```python
from build123d import *

# Parameters (mm, degrees)
EXTRUDE_1_DEPTH     = 30
CUT_EXTRUDE_1_DEPTH = 46.650848842
CUT_EXTRUDE_2_DEPTH = 46.650848842
FILLET_2_R          = 4
FILLET_3_R          = 3


with BuildPart() as part:
    # 草图1 → 凸台-拉伸1 (new body)
    with BuildSketch(Plane(origin=(0, 0, 0), x_dir=(0, 0, -1), z_dir=(1, 0, 0))):
        Polygon((0, 0), (0, -17.457543398), (0, -28), (3.576042669, -28), (20, -28), (20, -26), (3.746159887, -26), (2, -26), (2, -18.350485623), (2, 0), align=None)
    extrude(amount=EXTRUDE_1_DEPTH)

    # 草图3 → 切除-拉伸1 (cut, through all)
    with BuildSketch(Plane.XY):
        with BuildLine():
            Line((4, -12.5), (26, -12.5))
            ThreePointArc((26, -12.5), (28, -14.5), (26, -16.5))
            Line((26, -16.5), (4, -16.5))
            ThreePointArc((4, -16.5), (2, -14.5), (4, -12.5))
        make_face()
        with BuildLine():
            Line((4, -4.5), (26, -4.5))
            ThreePointArc((26, -4.5), (28, -6.5), (26, -8.5))
            Line((26, -8.5), (4, -8.5))
            ThreePointArc((4, -8.5), (2, -6.5), (4, -4.5))
        make_face()
    extrude(amount=-CUT_EXTRUDE_1_DEPTH, mode=Mode.SUBTRACT)

    # 草图4 → 切除-拉伸2 (cut, through all)
    with BuildSketch(Plane.XZ.offset(28)):
        with BuildLine():
            Line((4, -12.5), (26, -12.5))
            ThreePointArc((26, -12.5), (28.5, -15), (26, -17.5))
            Line((26, -17.5), (4, -17.5))
            ThreePointArc((4, -17.5), (1.5, -15), (4, -12.5))
        make_face()
    extrude(amount=-CUT_EXTRUDE_2_DEPTH, mode=Mode.SUBTRACT)

    # 圆角2
    fillet_2_edges = [part.edges().sort_by_distance(p)[0] for p in [
        (15, -28, 0),
    ]]
    fillet(fillet_2_edges, radius=FILLET_2_R)

    # 圆角3
    fillet_3_edges = [part.edges().sort_by_distance(p)[0] for p in [
        (15, -26, -2),
    ]]
    fillet(fillet_3_edges, radius=FILLET_3_R)


solid = part.part
```
Input: part model. Units: mm. Frame: model coordinates. A direction names the side the tool comes from. Give positions to 0.01 mm unless a question says otherwise; leave off trailing zeros. Write each loop counter-clockwise with the first axis right and the second up, starting at its lowest first coordinate (ties: lowest second). Pieces come first, ordered by that corner, then holes. Notation, with made-up numbers: (6, 74.5) - (10, 74.5) arc R22 cw to (10, 93.5) - close; hole circle Ø5 at (88, 22.25). An arc over 180 degrees is marked (long way). Write item = value, one per line. Start each with the question number.
1) Cut plane B-B (x = 5.25). Return loops of the section in (y, z).
2) Draft query along Z for faces 6 (the face through (15.21, -26.797, -1.141)), 7 (the face through (15, -16.5, -1)), 8 (the face through (15, -27, -12.5)). Return one class per face: pulls with the +Z half, pulls with the -Z half, needs draft (parallel to the pull), parting line crosses it, or undercut.
3) Cut plane A-A (z = -15). Return loops of the section in (x, y).
4) Material intervals for L1, parallel to Z at x = 8, y = -19.25; L2, parallel to Y at x = 13.25, z = -1.5; L3, parallel to Y at x = 6.5, z = -18.75, sorted ascending. Write a range as [from, to].
5) Pin query (flat end, axial travel): pin 1 (11.5 mm diameter, centred on x = 17, y = -14, fed in from -Z); pin 2 (2 mm diameter, centred on x = 20.5, z = -1, fed in from -Y); pin 3 (4.5 mm diameter, centred on x = 21.5, z = -13, fed in from +Y). Return the tip coordinate at first contact, or that it passes through.
6) Reachability of faces 1 (the face through (28, -6.5, -1)), 2 (the face through (1.5, -27, -15.1)), 3 (the face through (30, -19.1, -1.8)), 4 (the face through (0, -19.1, -1.8)), 5 (the face through (15, -26, -11)) from +Z, -Z, +X, -X, +Y, -Y: full face, straight path, thin tool, end or side. Return the list, or none.
7) Cut plane C-C (y = -14.5). Return loops of the section in (x, z).
8) Cut plane D-D (z = -11.25). Return loops of the section in (x, y), and give its area (3 significant figures).
Answers follow:
q1.outline = (-28, -20) - (-26, -20) - (-26, -17.5) - (-28, -17.5) - close; (-28, -12.5) - (-26, -12.5) - (-26, -5) arc R3 cw to (-23, -2) - (-16.5, -2) - (-16.5, 0) - (-24, 0) arc R4 ccw to (-28, -4) - close; (-12.5, -2) - (-8.5, -2) - (-8.5, 0) - (-12.5, 0) - close; (-4.5, -2) - (0, -2) - (0, 0) - (-4.5, 0) - close
q2.face_6 = pulls with the +Z half
q2.face_7 = needs draft
q2.face_8 = undercut
q3.outline = (0, -28) - (1.5, -28) - (1.5, -26) - (0, -26) - close; (28.5, -28) - (30, -28) - (30, -26) - (28.5, -26) - close
q4.L1 = [-2, 0]
q4.L2 = [-27.12, -16.5], [-12.5, -8.5], [-4.5, 0]
q4.L3 = [-28, -26]
q5.pin_1 = -2
q5.pin_2 = -27.46
q5.pin_3 = -26
q6.face_1 = +Z, -Z
q6.face_2 = +Y, -Y
q6.face_3 = +Z, -Z, +X, +Y, -Y
q6.face_4 = +Z, -Z, -X, +Y, -Y
q6.face_5 = -Z, +X, -X, +Y
q7.outline = (0, -2) - (2, -2) - (2, 0) - (0, 0) - close; (28, -2) - (30, -2) - (30, 0) - (28, 0) - close
q8.outline = (0, -28) - (30, -28) - (30, -26) - (0, -26) - close
q8.area = 60.0 mm^2
